The listing builds one solid part. Answer for the finished solid, in the listing's coordinates (mm). Face numbers are marked on the shaded views. Give positions to 0.01 mm unless a question says otherwise; leave off trailing zeros. Write each loop counter-clockwise with the first axis right and the second up, starting at its lowest first coordinate (ties: lowest second). Pieces come first, ordered by that corner, then holes. Notation, with made-up numbers: (-13.75, 29.25) - (-3.75, 29.25) arc R9 ccw to (-3.75, 46.25) - close; hole circle Ø7 at (21.5, 34). An arc over 180 degrees is marked (long way). One line per question, with ' | ' between items. Start each with the question number.
1. Given P1, Ø6, axis at y = 330, z = 6.5, coming from the -X side; P2, Ø5.5, axis at x = 44.45, y = 171.45, coming from the +Z side, each flat-ended and moving along its own axis, determine where each tip first touches the part or whether it passes through.
2. Find the intervals of material crossed by L1, parallel to Y at x = 44, z = 20; L2, parallel to X at y = 336.55, z = 17.5; L3, parallel to Y at x = 46, z = 9.5, in increasing order. Write a range as from..to.
3. A cutting plane is placed at A-A (y = 336.55). Determine the outline of the cut face in (x, z), then the cut area to 3 significant figures.
4. A cutting plane is placed at B-B (x = 44.45). Determine the outline of the cut face in (y, z), then the cut area to 3 significant figures.
5. The mould has two halves that part along X. Classify the marked faces 1, 2 and 3: +X half, -X half, draft (parallel to the pull), parting line (faces both ways), or undercut.
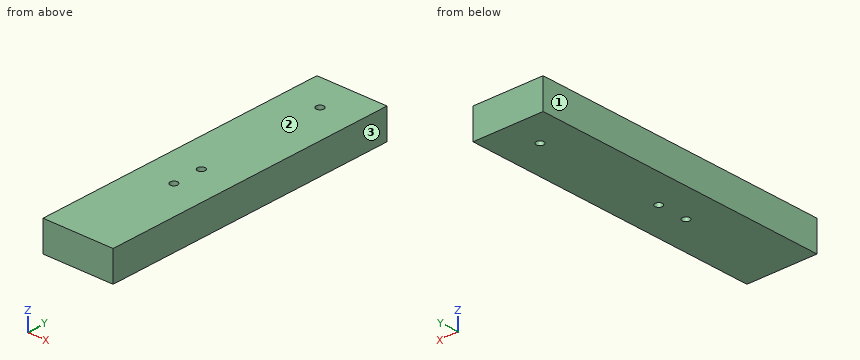
```python
from build123d import *

# Parameters (mm, degrees)
SKETCH1_W           = 88.9
SKETCH1_H           = 381
BOSS_EXTRUDE1_DEPTH = 38.1
SKETCH2_R           = 4.7625
CUT_EXTRUDE1_DEPTH  = 394.08500353
SKETCH3_R           = 4.7625
CUT_EXTRUDE2_DEPTH  = 394.08500353
SKETCH4_R           = 4.7625
CUT_EXTRUDE3_DEPTH  = 394.08500353


with BuildPart() as part:
    # Sketch1 → Boss-Extrude1 (new body)
    with BuildSketch(Plane.XY):
        with Locations((44.45, 190.5)):
            Rectangle(SKETCH1_W, SKETCH1_H)
    extrude(amount=BOSS_EXTRUDE1_DEPTH)

    # Sketch2 → Cut-Extrude1 (cut, through all)
    with BuildSketch(Plane.XY.offset(38.1)):
        with Locations((44.45, 133.35)):
            Circle(SKETCH2_R)
    extrude(amount=-CUT_EXTRUDE1_DEPTH, mode=Mode.SUBTRACT)

    # Sketch3 → Cut-Extrude2 (cut, through all)
    with BuildSketch(Plane.XY.offset(38.1)):
        with Locations((44.45, 336.55)):
            Circle(SKETCH3_R)
    extrude(amount=-CUT_EXTRUDE2_DEPTH, mode=Mode.SUBTRACT)

    # Sketch4 → Cut-Extrude3 (cut, through all)
    with BuildSketch(Plane.XY.offset(38.1)):
        with Locations((44.45, 171.45)):
            Circle(SKETCH4_R)
    extrude(amount=-CUT_EXTRUDE3_DEPTH, mode=Mode.SUBTRACT)


solid = part.part
```
Determined:
1) P1: x = 0 | P2: through
2) L1: 0..128.61, 138.09..166.71, 176.19..331.81, 341.29..381 | L2: 0..39.69, 49.21..88.9 | L3: 0..128.85, 137.85..166.95, 175.95..332.05, 341.05..381
3) outline: (0, 0) - (39.69, 0) - (39.69, 38.1) - (0, 38.1) - close; (49.21, 0) - (88.9, 0) - (88.9, 38.1) - (49.21, 38.1) - close | area: 3,020 mm2
4) outline: (0, 0) - (128.59, 0) - (128.59, 38.1) - (0, 38.1) - close; (138.11, 0) - (166.69, 0) - (166.69, 38.1) - (138.11, 38.1) - close; (176.21, 0) - (331.79, 0) - (331.79, 38.1) - (176.21, 38.1) - close; (341.31, 0) - (381, 0) - (381, 38.1) - (341.31, 38.1) - close | area: 13,400 mm2
5) face 1: -X half | face 2: draft | face 3: +X half
